from build123d import *

# Parameters (mm, degrees)
BASE_EXTRUDE_DEPTH = 3


with BuildPart() as part:
    # Sketch1 → Base-Extrude (new body)
    with BuildSketch(Plane.XY):
        with BuildLine():
            Line((796.067430824, -94.790628806), (796.067430824, -97.790628806))
            Line((796.067430824, -97.790628806), (791.272591236, -97.790628806))
            ThreePointArc((791.272591236, -97.790628806), (789.599137263, -99.319974572), (788.471131564, -101.286430728))
            ThreePointArc((788.471131564, -101.286430728), (787.733624184, -104.495988694), (788.471131564, -107.705546661))
            ThreePointArc((788.471131564, -107.705546661), (789.599137263, -109.672002816), (791.272591236, -111.201348582))
            Line((791.272591236, -111.201348582), (796.067430824, -111.201348582))
            Line((796.067430824, -111.201348582), (796.067430824, -114.201348582))
            Line((796.067430824, -114.201348582), (791.272591236, -114.201348582))
            Line((791.272591236, -114.201348582), (792.051319906, -120.205546661))
            Line((792.051319906, -120.205546661), (795.668694327, -120.205546661))
            Line((795.668694327, -120.205546661), (795.668694327, -123.205546661))
            Line((795.668694327, -123.205546661), (785.561028396, -123.205546661))
            ThreePointArc((785.561028396, -123.205546661), (785.308371949, -125.550343576), (786.768988057, -127.401966768))
            ThreePointArc((786.768988057, -127.401966768), (791.730710774, -128.428848688), (796.763839141, -127.845069923))
            Line((796.763839141, -127.845069923), (796.763839141, -137.690530558))
            ThreePointArc((796.763839141, -137.690530558), (797.399275262, -139.224609057), (798.933353761, -139.860045178))
            Line((798.933353761, -139.860045178), (801.559237467, -139.860045178))
            ThreePointArc((801.559237467, -139.860045178), (803.122225358, -139.173347979), (803.657482492, -137.552242187))
            Line((803.657482492, -137.552242187), (803.657482492, -130.563057952))
            Line((803.657482492, -130.563057952), (811.531636536, -129.07193908))
            Line((811.531636536, -129.07193908), (811.531636536, -119.995988694))
            Line((811.531636536, -119.995988694), (801.531636536, -119.995988694))
            Line((801.531636536, -119.995988694), (801.531636536, -116.995988694))
            Line((801.531636536, -116.995988694), (811.531636536, -116.995988694))
            Line((811.531636536, -116.995988694), (811.531636536, -95.495988694))
            Line((811.531636536, -95.495988694), (797.954990923, -95.495988694))
            Line((797.954990923, -95.495988694), (797.954990923, -94.995988694))
            Line((797.954990923, -94.995988694), (797.954990923, -91.995988694))
            Line((797.954990923, -91.995988694), (801.531636536, -91.995988694))
            Line((801.531636536, -91.995988694), (801.531636536, -88.995988694))
            Line((801.531636536, -88.995988694), (811.531636536, -88.995988694))
            Line((811.531636536, -88.995988694), (811.531636536, -79.920038308))
            Line((811.531636536, -79.920038308), (803.657482492, -78.428919436))
            Line((803.657482492, -78.428919436), (803.657482492, -71.439735201))
            ThreePointArc((803.657482492, -71.439735201), (803.122225358, -69.818629409), (801.559237467, -69.131932211))
            Line((801.559237467, -69.131932211), (798.933353761, -69.131932211))
            ThreePointArc((798.933353761, -69.131932211), (797.399275262, -69.767368331), (796.763839141, -71.30144683))
            Line((796.763839141, -71.30144683), (796.763839141, -81.146907465))
            ThreePointArc((796.763839141, -81.146907465), (791.730710774, -80.5631287), (786.768988057, -81.590010621))
            ThreePointArc((786.768988057, -81.590010621), (785.308371949, -83.441633812), (785.561028396, -85.786430728))
            Line((785.561028396, -85.786430728), (795.668694327, -85.786430728))
            Line((795.668694327, -85.786430728), (795.668694327, -88.786430728))
            Line((795.668694327, -88.786430728), (792.051319906, -88.786430728))
            Line((792.051319906, -88.786430728), (791.272591236, -94.790628806))
            Line((791.272591236, -94.790628806), (796.067430824, -94.790628806))
        make_face()
    extrude(amount=BASE_EXTRUDE_DEPTH)


solid = part.part
Source: CAD feature listing. Evaluate the final solid. Frame: model axes, mm. A direction names the side the tool comes from. Coordinates: 2 decimals unless noted, no trailing zeros. Loops run counter-clockwise (first coordinate to the right, second up) from the corner with the lowest first, then second, coordinate; pieces in that order, holes last. Notation, with made-up numbers: (77.5, 57) - (94.5, 57) arc R27 ccw to (94.5, 77) - close; hole circle Ø4 at (-11.75, 58.25). An arc over 180 degrees is marked (long way). One line per question, with ' | ' between items.
1) Section A-A, the plane x = 800.25. Return loops of the section in (y, z), then the cut area to 3 significant figures.
Report:
outline: (-139.86, 0) - (-95.5, 0) - (-95.5, 3) - (-139.86, 3) - close; (-92, 0) - (-69.13, 0) - (-69.13, 3) - (-92, 3) - close | area: 202 mm²
2) First-contact query: P1, Ø0.9, axis at x = 808.5, z = 2, coming from the -Y side; P2, Ø1.5, axis at y = -92, z = 2.5, coming from the +X side; P3, Ø1.5, axis at x = 805, z = 1.5, coming from the -Y side. Flat tips, straight axial feed; report the tip coordinate or a pass-through.
Report:
P1: stops at y = -129.73 | P2: stops at x = 801.53 | P3: stops at y = -130.45
3) Set-up query: faces 1 (the face through (811.532, -106, 1)), 2 (the face through (801.532, -91, 1)), 3 (the face through (795.669, -122, 1)). Return all of +Z, -Z, +X, -X, +Y, -Y with unobstructed straight access to the full face (end or side cutting, diameter ignored); none if empty.
Report:
face 1: +Z, -Z, +X, +Y, -Y | face 2: +Z, -Z, +X | face 3: +Z, -Z, -X
4) Section B-B, the plane x = 789.5. Return loops of the section in (y, z).
Report:
outline: (-128.17, 0) - (-123.21, 0) - (-123.21, 3) - (-128.17, 3) - close; (-109.55, 0) - (-99.45, 0) - (-99.45, 3) - (-109.55, 3) - close; (-85.79, 0) - (-80.82, 0) - (-80.82, 3) - (-85.79, 3) - close
5) Line query: line 1 along Y through (x, z) = (799, 1.1); line 2 along Y through (x, z) = (808.5, 0.2); line 3 along X through (y, z) = (-75, 1.15). Output: solid intervals per line, ascending.
Report:
line 1: y = -139.86 to -95.5, -92 to -69.13 | line 2: y = -129.65 to -120, -117 to -95.5, -89 to -79.35 | line 3: x = 796.76 to 803.66
6) Section C-C, the plane y = -112.5. Return loops of the section in (x, z).
Report:
outline: (796.07, 0) - (811.53, 0) - (811.53, 3) - (796.07, 3) - close
7) Section D-D, the plane x = 806.75. Return loops of the section in (y, z).
Report:
outline: (-129.98, 0) - (-120, 0) - (-120, 3) - (-129.98, 3) - close; (-117, 0) - (-95.5, 0) - (-95.5, 3) - (-117, 3) - close; (-89, 0) - (-79.01, 0) - (-79.01, 3) - (-89, 3) - close
8) Pull-direction query (Y, two-part tool) for faces 4 (the face through (807.539, -129.828, 1.479)), 5 (the face through (789.58, -109.65, 1.48)), 6 (the face through (796.764, -76, 1)); classes: released by +Y, released by -Y, zero draft, split by the parting line, or undercut.
Report:
face 4: released by -Y | face 5: undercut | face 6: zero draft
